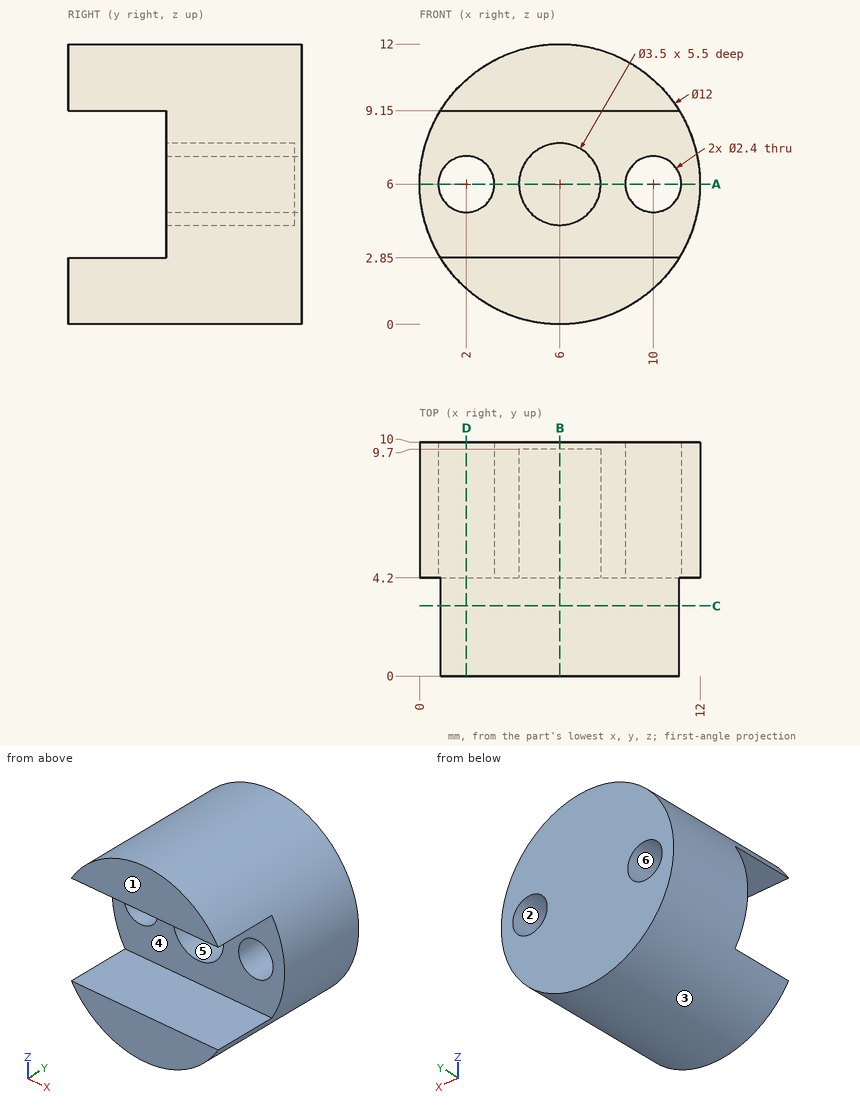
Can you work these out from the drawing? Everything is in mm from the part's minimum corner. A direction names the side the tool comes from. Give positions to 0.01 mm unless a question says otherwise; leave off trailing zeros. Loops run counter-clockwise (first coordinate to the right, second up) from the corner with the lowest first, then second, coordinate; pieces in that order, holes last. Notation, with made-up numbers: M 2.25,39.25 L 30.25,39.25 A30 ccw 30.25,64.25 Z; hole C 41.25,58.25 d2. An arc over 180 degrees is marked long. Use CSV: the item, a comma, the result in double quotes. Start each with the question number.
1. On a 3-axis mill with a long thin cutter (end or side, diameter ignored), from which of +Z, -Z, +X, -X, +Y, -Y can I reach the whole of each face in a straight line? I mean the marked faces 4, 5 and 6. Say none if no direction works.
2. Imagine slicing it at B-B, the plane x = 6. Write out the boundary of the cut face in (y, z).
3. If I drill on L1, parallel to X at y = 8.15, z = 6; L2, parallel to X at y = 7.5, z = 5.5; L3, parallel to Y at x = 10, z = 3, over which ranges is the centre line in solid material (lowest first)?
4. Imagine slicing it at C-C, the plane y = 3. Write out the boundary of the cut face in (x, z).
5. Imagine slicing it at D-D, the plane x = 2. Write out the boundary of the cut face in (y, z), plus the area to 3 significant figures.
6. For P1, Ø3, axis at x = 5, z = 7.5, coming from the -Y side; P2, Ø5, axis at x = 3, y = 3, coming from the -Z side; P3, Ø5, axis at y = 7.5, z = 8, coming from the +X side; P4, Ø5, axis at y = 1.5, z = 7, coming from the +X side, each with a flat end and sliding along its axis, tell me the tip position at first contact or that it passes through.
7. Imagine slicing it at A-A, the plane z = 6. Write out the boundary of the cut face in (x, y).
8. If we mould it in two halves opening along Z, with no side actions, what happens to the marked faces 1, 2 and 3? For each: released by +Z, released by -Z, zero draft, split by the parting line, or undercut.
Response values:
1,face 4,"+X, -X, -Y"
1,face 5,"-Y"
1,face 6,"+Y, -Y"
2,outline,"M 0,0 L 10,0 L 10,12 L 0,12 L 0,9.15 L 4.2,9.15 L 4.2,7.75 L 9.7,7.75 L 9.7,4.25 L 4.2,4.25 L 4.2,2.85 L 0,2.85 Z"
3,L1,"0 to 0.8, 3.2 to 4.25, 7.75 to 8.8, 11.2 to 12"
3,L2,"0.02 to 0.91, 3.09 to 4.32, 7.68 to 8.91, 11.09 to 11.98"
3,L3,"4.2 to 10"
4,outline,"M 0.89,2.85 A6 ccw 11.11,2.85 Z; M 0.89,9.15 L 11.11,9.15 A6 ccw Z"
5,outline,"M 0,1.53 L 10,1.53 L 10,4.8 L 4.2,4.8 L 4.2,2.85 L 0,2.85 Z; M 0,9.15 L 4.2,9.15 L 4.2,7.2 L 10,7.2 L 10,10.47 L 0,10.47 Z"
5,area,"49.1 mm^2"
6,P1,"y = 4.2"
6,P2,"z = 0.02"
6,P3,"x = 12"
6,P4,"x = 11.11"
7,outline,"M 0,4.2 L 0.8,4.2 L 0.8,10 L 0,10 Z; M 3.2,4.2 L 4.25,4.2 L 4.25,9.7 L 7.75,9.7 L 7.75,4.2 L 8.8,4.2 L 8.8,10 L 3.2,10 Z; M 11.2,4.2 L 12,4.2 L 12,10 L 11.2,10 Z"
8,face 1,"zero draft"
8,face 2,"undercut"
8,face 3,"split by the parting line"
